Geometry: see drawing. Coordinates: mm, zero at the bounding-box minimum. A direction names the side the tool comes from. Round coordinates to 2 decimals unless told otherwise and drop trailing zeros. Write each loop counter-clockwise with the first axis right and the second up, starting at its lowest first coordinate (ties: lowest second). Pieces come first, ordered by that corner, then holes. Notation, with made-up numbers: (-40, 28) - (-14, 28) arc R6 ccw to (-14, 39) - close; hole circle Ø2 at (-24.5, 53). An arc over 180 degrees is marked (long way). Use a Markdown table: item, result. Add a question column.
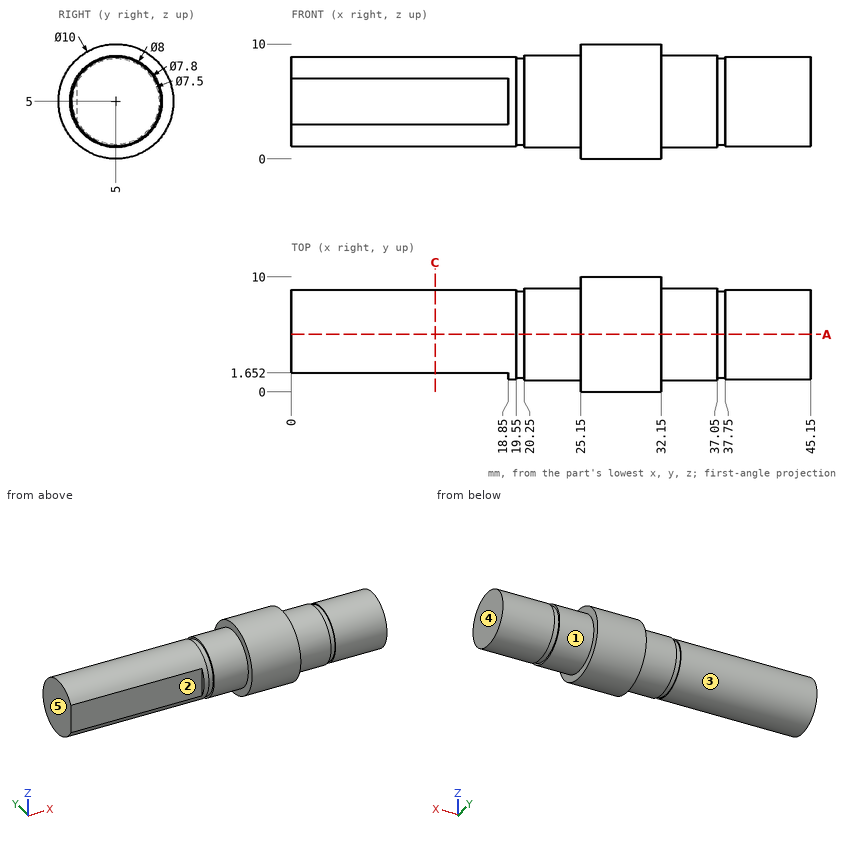
1) Pin query (flat end, axial travel): P1, Ø1.5, axis at x = 6.5, z = 1, coming from the +Y side; P2, Ø2, axis at x = 8.5, z = 5.5, coming from the -Y side; P3, Ø5, axis at x = 6, y = 2.5, coming from the +Z side. Return the tip coordinate at first contact, or that it passes through.
2) Set-up query: the marked faces 1, 2, 3, 4 and 5. Return all of +Z, -Z, +X, -X, +Y, -Y with unobstructed straight access to the full face (end or side cutting, diameter ignored); none if empty.
3) Section A-A, the plane y = 5. Return the cut outline in (x, z).
4) Material intervals for L1, parallel to X at y = 7, z = 1.75; L2, parallel to X at y = 8, z = 8.5; L3, parallel to Z at x = 28, y = 2, sorted ascending. Write a range as from..to.
5) Section C-C, the plane x = 12.5. Return the cut outline in (y, z).
Output values:
| question | item | result |
|---|---|---|
| 1 | P1 | stops at y = 7.16 |
| 1 | P2 | stops at y = 1.65 |
| 1 | P3 | stops at z = 8.9 |
| 2 | face 1 | +X |
| 2 | face 2 | +Z, -Z, -X, -Y |
| 2 | face 3 | -X |
| 2 | face 4 | +Z, -Z, +X, +Y, -Y |
| 2 | face 5 | +Z, -Z, -X, +Y, -Y |
| 3 | outline | (0, 1.1) - (19.55, 1.1) - (19.55, 1.25) - (20.25, 1.25) - (20.25, 1) - (25.15, 1) - (25.15, 0) - (32.15, 0) - (32.15, 1) - (37.05, 1) - (37.05, 1.25) - (37.75, 1.25) - (37.75, 1.1) - (45.15, 1.1) - (45.15, 8.9) - (37.75, 8.9) - (37.75, 8.75) - (37.05, 8.75) - (37.05, 9) - (32.15, 9) - (32.15, 10) - (25.15, 10) - (25.15, 9) - (20.25, 9) - (20.25, 8.75) - (19.55, 8.75) - (19.55, 8.9) - (0, 8.9) - close |
| 4 | L1 | x = 0..19.55, 20.25..37.05, 37.75..45.15 |
| 4 | L2 | x = 25.15..32.15 |
| 4 | L3 | z = 1..9 |
| 5 | outline | (1.65, 3) arc R3.9 ccw (long way) to (1.65, 7) - close |
